Here's how the part is built. I have some questions about the finished solid (model axes, mm). A direction names the side the tool comes from. Coordinates: 2 decimals unless noted, no trailing zeros. Answer in a Markdown table with one row per item. Add a question column.
Item 1: Thinking about a two-plate mould opening in X: for faces 1 (the cylindrical face through (21.7, 35.3, 15.8)), 2 (the flat face through (22, 39, 19.05)), which applies, +X half, -X half, draft (parallel to the pull), parting line (faces both ways), or undercut?
Item 2: On a 3-axis mill with a long thin cutter (end or side, diameter ignored), from which of +Z, -Z, +X, -X, +Y, -Y can I reach the whole of each face in a straight line? I mean faces 3 (the flat face through (6.35, -20, 5)), 4 (the flat face through (0, 45, 19.05)), 5 (the flat face through (-7, 1, 0)), 6 (the flat face through (0, 31.75, 6)), 7 (the cylindrical face through (-48.026, -2.301, 15.831)). Say none if no direction works.
Item 3: If I drill on line 1 along Y through (x, z) = (42, 13.5); line 2 along X through (y, z) = (38.5, 7.5); line 3 along Z through (x, y) = (0, 44.5), over which ranges is the centre line in solid material (lowest first)? Write a range as from..to.
Item 4: Will these pins go through, and if not, where does the flat tip stop? pin 1 Ø6.5 at (y, z) = (-31.5, 9) entering from -X; pin 2 Ø1 at (y, z) = (-22, 6) entering from +X; pin 3 Ø4.5 at (x, z) = (0, 6.35) entering from +Y.
Item 5: I want a section at A-A (z = 17.25). Count the separate pieces of the cut face and the enclosed holes in it, plus the area to 3 significant figures.
```python
from build123d import *

# Parameters (mm, degrees)
F0_R      = 50.8
F1_DEPTH  = 12.7
F3_R      = 38.1
F4_DEPTH  = 6.35
F6_W      = 12.7
F6_H      = 83.8771756418
F7_DEPTH  = 25.4
F9_R      = 3.81
F10_DEPTH = 41.656
F11_R     = 3.7810776449
F12_DEPTH = 6.35


# Not quite as in the source:
# - a fillet or chamfer that OpenCascade refuses, or shapes differently, is made with other operations: its cross-section is extruded or revolved along the edge and cut away or added


with BuildPart() as f1:
    # F0 (on Top) → F1 (new body)
    with BuildSketch(Plane.XY):
        Circle(F0_R)
    extrude(amount=F1_DEPTH)

    # F2: fillet of radius 25.4 on 1 edges, made by hand

    # F2_s1 → F2_t2 (revolve, cut)
    with BuildSketch(Plane.XZ):
        with BuildLine():
            ThreePointArc((50.8, 12.7), (41.5029547439, 3.4029547439), (28.8029547439, 0))
            Line((28.8029547439, 0), (28.8029547439, -0.508))
            Line((28.8029547439, -0.508), (50.8, -0.508))
            Line((50.8, -0.508), (51.308, 0))
            ThreePointArc((51.308, 0), (51.308, 6.35), (51.2399409051, 12.446))
            Line((51.2399409051, 12.446), (50.8, 12.7))
        make_face()
    revolve(axis=Axis((0, 0, 0), (0, 0, 1)), mode=Mode.SUBTRACT)

    # F3 (on face) → F4 (cut)
    with BuildSketch(Plane.XY.offset(12.7)):
        Circle(F3_R)
    extrude(amount=-F4_DEPTH, mode=Mode.SUBTRACT)

    # F5: fillet of radius 114.3 on 1 edges, made by hand

    # F5_s1 → F5_t2 (revolve)
    with BuildSketch(Plane.XZ):
        with BuildLine():
            ThreePointArc((38.1, 12.7), (19.5828933773, 7.948680132), (0.5328933773, 6.35))
            Line((0.5328933773, 6.35), (38.1, 6.35))
            Line((38.1, 6.35), (38.1, 12.7))
        make_face()
    revolve(axis=Axis((0, 0, 6.35), (0, 0, 1)))

    # F6 (on face) → F7 (cut)
    with BuildSketch(Plane.XY.offset(12.7)):
        with Locations((0, -30.5251618847)):
            Rectangle(F6_W, F6_H)
    extrude(amount=-F7_DEPTH, mode=Mode.SUBTRACT)

    # F9 (on offset) → F10 (cut)
    with BuildSketch(Plane.XZ.offset(-73.406)):
        with Locations((0, 6.35)):
            Circle(F9_R)
    extrude(amount=F10_DEPTH, mode=Mode.SUBTRACT)

    # F11 (on face) → F12 (join)
    with BuildSketch(Plane.XY.offset(12.7)):
        with Locations((-45.025870204, 0)):
            Circle(F11_R)
        with Locations((-38.9935474241, -22.512935102)):
            Circle(F11_R)
        with Locations((-22.512935102, -38.9935474241)):
            Circle(F11_R)
        with Locations((22.512935102, -38.9935474241)):
            Circle(F11_R)
        with Locations((38.9935474241, -22.512935102)):
            Circle(F11_R)
        with Locations((45.025870204, 0)):
            Circle(F11_R)
        with Locations((38.9935474241, 22.512935102)):
            Circle(F11_R)
        with Locations((22.512935102, 38.9935474241)):
            Circle(F11_R)
        with Locations((0, 45.025870204)):
            Circle(F11_R)
        with Locations((-22.512935102, 38.9935474241)):
            Circle(F11_R)
        with Locations((-38.9935474241, 22.512935102)):
            Circle(F11_R)
    extrude(amount=F12_DEPTH)


solid = f1.part
```
Values follow:
| question | item | result |
|---|---|---|
| 1 | face 1 | undercut |
| 1 | face 2 | draft |
| 2 | face 3 | +Z, -Z, -Y |
| 2 | face 4 | +Z, +X, -X, +Y, -Y |
| 2 | face 5 | -Z, +X, -X, +Y, -Y |
| 2 | face 6 | +Y |
| 2 | face 7 | +Z |
| 3 | line 1 | y = -24.81..-20.22, -2.27..2.27, 20.22..24.81 |
| 3 | line 2 | x = -26.65..-3.63, 3.63..26.65 |
| 3 | line 3 | z = 10.16..19.05 |
| 4 | pin 1 | stops at x = -40.51 |
| 4 | pin 2 | stops at x = 40.19 |
| 4 | pin 3 | stops at y = 31.75 |
| 5 | separate pieces | 11 |
| 5 | enclosed holes | 0 |
| 5 | area | 494 mm^2 |
